Part print with two shaded views. Sizes in mm from the minimum x, y, z corner. Round coordinates to 2 decimals unless told otherwise and drop trailing zeros. Loops run counter-clockwise (first coordinate to the right, second up) from the corner with the lowest first, then second, coordinate; pieces in that order, holes last. Notation, with made-up numbers: M 56,-30.5 L 104,-30.5 A6 cw 104,-22.5 Z; hole C 21,-20.5 d3. An arc over 180 degrees is marked long. Answer as CSV lines item,"result". Start each with the question number.
Item 1: Wall check: line 1 (Z direction, x = 23, y = 1.5); line 2 (Y direction, x = 41, z = 22.65); line 3 (Z direction, x = 35, y = 18.75). Give the ranges that are in metal, low to high.
Item 2: Band-saw the part on D-D (x = 18). Give the cut face in (y, z).
Item 3: Band-saw the part on A-A (z = 13.5). Give the cut face in (x, y), and give its area (3 significant figures).
Item 4: Drop flat-ended pins along their axis: pin 1 Ø10 at (x, z) = (38.5, 6) entering from -Y; pin 2 Ø2 at (x, z) = (35, 22) entering from -Y; pin 3 Ø6 at (x, y) = (31.5, 11.5) entering from -Z. Give the stop position or say it passes through.
Item 5: Band-saw the part on B-B (x = 4). Give the cut face in (y, z), and give its area (3 significant figures).
Item 6: Mould opens along Z. For the marked faces 1, 2 and 3 say: pulls with the +Z half, pulls with the -Z half, needs draft (parallel to the pull), parting line crosses it, or undercut.
Item 7: Band-saw the part on C-C (y = 21). Give the cut face in (x, z), and give its area (3 significant figures).
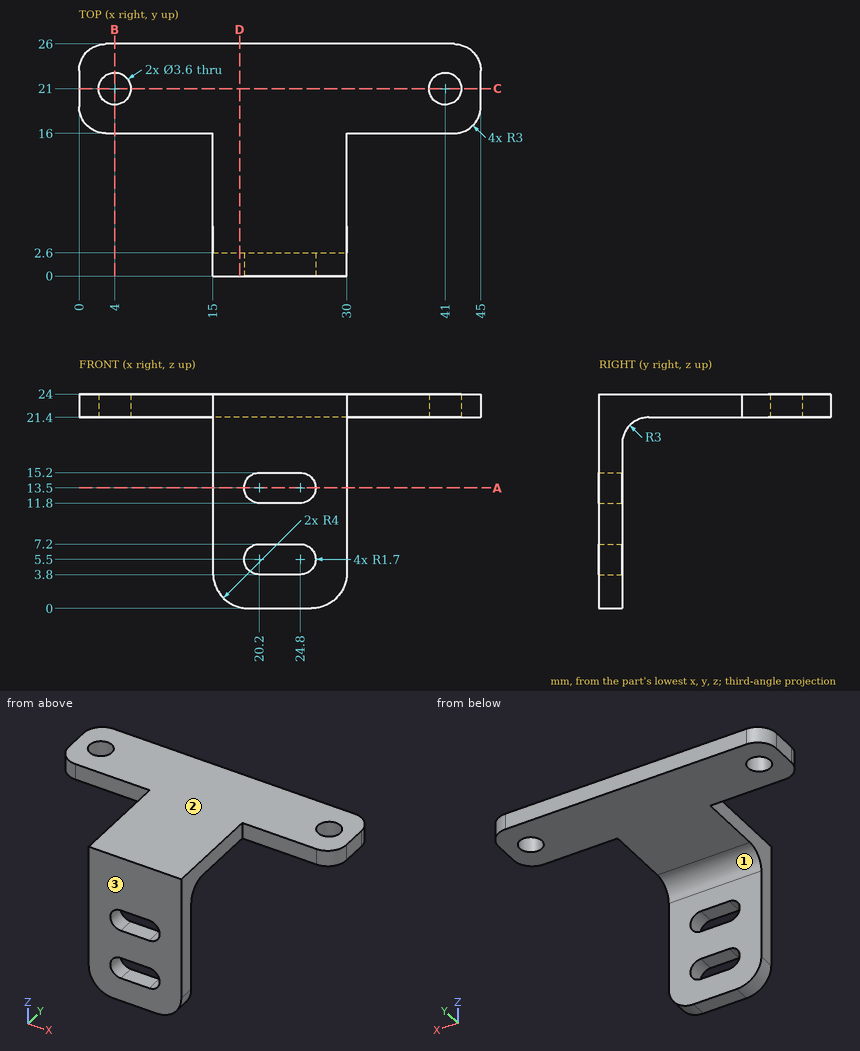
Answer block:
1,line 1,"z = 0 to 3.8, 7.2 to 11.8, 15.2 to 24"
1,line 2,"y = 16 to 19.2, 22.8 to 26"
1,line 3,"z = 21.4 to 24"
2,outline,"M 0,0.13 L 2.6,0.13 L 2.6,18.4 A3 cw 5.6,21.4 L 26,21.4 L 26,24 L 0,24 Z"
3,outline,"M 15,0 L 18.5,0 L 18.5,2.6 L 15,2.6 Z; M 26.5,0 L 30,0 L 30,2.6 L 26.5,2.6 Z"
3,area,"18.2 mm^2"
4,pin 1,"passes through"
4,pin 2,"stops at y = 16"
4,pin 3,"stops at z = 21.4"
5,outline,"M 16,21.4 L 19.2,21.4 L 19.2,24 L 16,24 Z; M 22.8,21.4 L 26,21.4 L 26,24 L 22.8,24 Z"
5,area,"16.6 mm^2"
6,face 1,"pulls with the -Z half"
6,face 2,"pulls with the +Z half"
6,face 3,"needs draft"
7,outline,"M 0,21.4 L 2.2,21.4 L 2.2,24 L 0,24 Z; M 5.8,21.4 L 39.2,21.4 L 39.2,24 L 5.8,24 Z; M 42.8,21.4 L 45,21.4 L 45,24 L 42.8,24 Z"
7,area,"98.3 mm^2"
